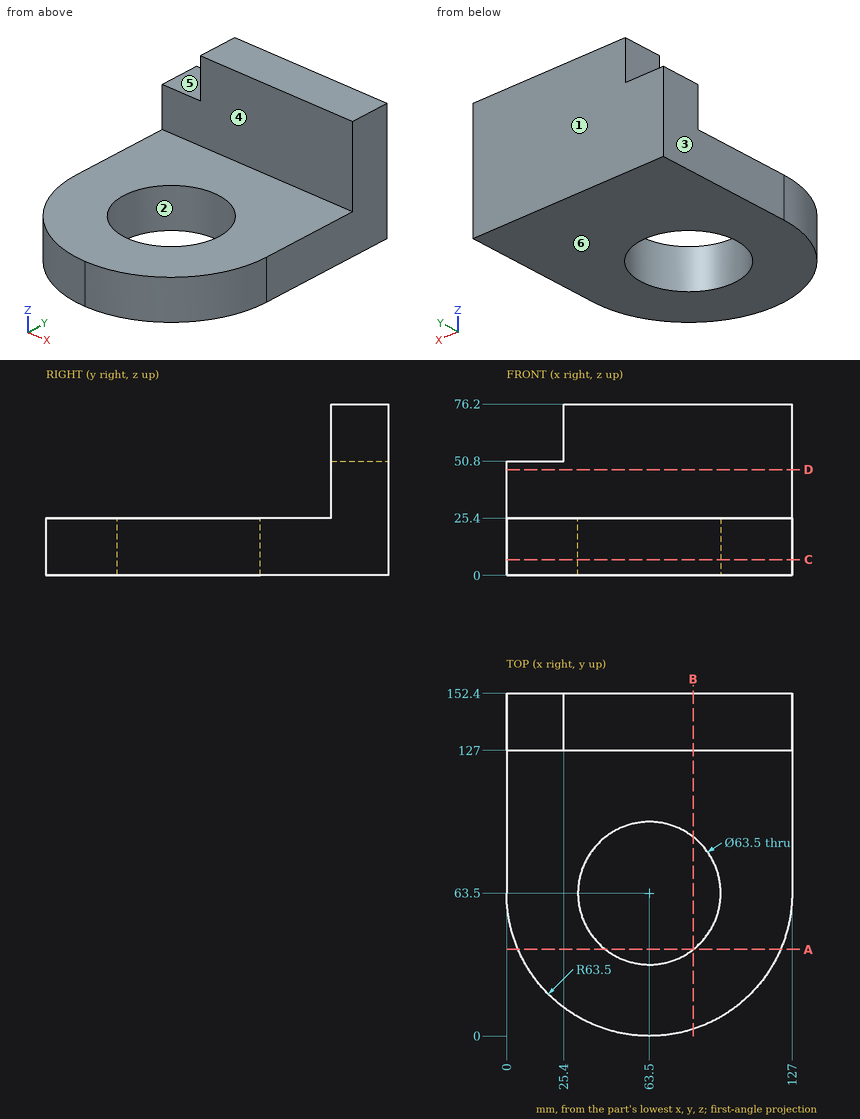
Study the drawing (mm; zero at the part's minimum x, y, z) and answer. A direction names the side the tool comes from. Coordinates: 2 decimals unless noted, no trailing zeros. Loops run counter-clockwise (first coordinate to the right, second up) from the corner with the lowest first, then second, coordinate; pieces in that order, holes last. Notation, with made-up numbers: M 22,33 L 38,33 A32 ccw 38,61 Z; hole C 47.5,28 d8. An arc over 180 degrees is marked long. Answer in a Markdown table with one row per item.
1) Given pin 1 (8 mm diameter, centred on y = 53, z = 15.5, fed in from -X); pin 2 (1.5 mm diameter, centred on x = 103, z = 16.5, fed in from -Y); pin 3 (20.5 mm diameter, centred on x = 14.5, y = 133.5, fed in from +Z), each flat-ended and moving along its own axis, determine where each tip first touches the part or whether it passes through.
Answers below:
| item | result |
|---|---|
| pin 1 | x = 0.33 |
| pin 2 | y = 13.19 |
| pin 3 | z = 50.8 |
2) Find section B-B (x = 83). Determine the outline of the cut face in (y, z).
Answers below:
| item | result |
|---|---|
| outline | M 3.07,0 L 38.44,0 L 38.44,25.4 L 3.07,25.4 Z; M 88.56,0 L 152.4,0 L 152.4,76.2 L 127,76.2 L 127,25.4 L 88.56,25.4 Z |
3) Determine the mould class of the marked faces 1, 2 and 3 for opening direction X: released by +X, released by -X, zero draft, split by the parting line, or undercut.
Answers below:
| item | result |
|---|---|
| face 1 | zero draft |
| face 2 | undercut |
| face 3 | released by -X |
4) Which of the six approach directions +Z, -Z, +X, -X, +Y, -Y give full straight-line access (tool end or side, diameter ignored) to the marked faces 4, 5 and 6?
Answers below:
| item | result |
|---|---|
| face 4 | +Z, +X, -X, -Y |
| face 5 | +Z, -X, +Y, -Y |
| face 6 | -Z, +X, -X, +Y, -Y |
5) Find section C-C (z = 7). Determine the outline of the cut face in (x, y).
Answers below:
| item | result |
|---|---|
| outline | M 0,63.5 A63.5 ccw 63.5,0 A63.5 ccw 127,63.5 L 127,152.4 L 0,152.4 Z; hole C 63.5,63.5 d63.5 |
6) Find the intervals of material crossed by probe 1 along Y at (x, z) = (63, 12); probe 2 along X at (y, z) = (63, 13); probe 3 along Y at (x, z) = (38, 10.5), in increasing order.
Answers below:
| item | result |
|---|---|
| probe 1 | 0 to 31.75, 95.25 to 152.4 |
| probe 2 | 0 to 31.75, 95.25 to 127 |
| probe 3 | 5.35 to 44.58, 82.42 to 152.4 |
7) Find section D-D (z = 47). Determine the outline of the cut face in (x, y).
Answers below:
| item | result |
|---|---|
| outline | M 0,127 L 127,127 L 127,152.4 L 0,152.4 Z |
8) Find section A-A (y = 38.5). Determine the outline of the cut face in (x, z), then the cut area to 3 significant figures.
Answers below:
| item | result |
|---|---|
| outline | M 5.13,0 L 43.93,0 L 43.93,25.4 L 5.13,25.4 Z; M 83.07,0 L 121.87,0 L 121.87,25.4 L 83.07,25.4 Z |
| area | 1,970 mm^2 |
